Study the drawing (mm; zero at the part's minimum x, y, z) and answer. A direction names the side the tool comes from. Coordinates: 2 decimals unless noted, no trailing zeros. Loops run counter-clockwise (first coordinate to the right, second up) from the corner with the lowest first, then second, coordinate; pieces in that order, holes last. Notation, with made-up numbers: (70.5, 18) - (75.5, 18) arc R16 ccw to (75.5, 29) - close; hole circle Ø4 at (88, 33). An arc over 180 degrees is marked (long way). Use one line per item in the form item = value.
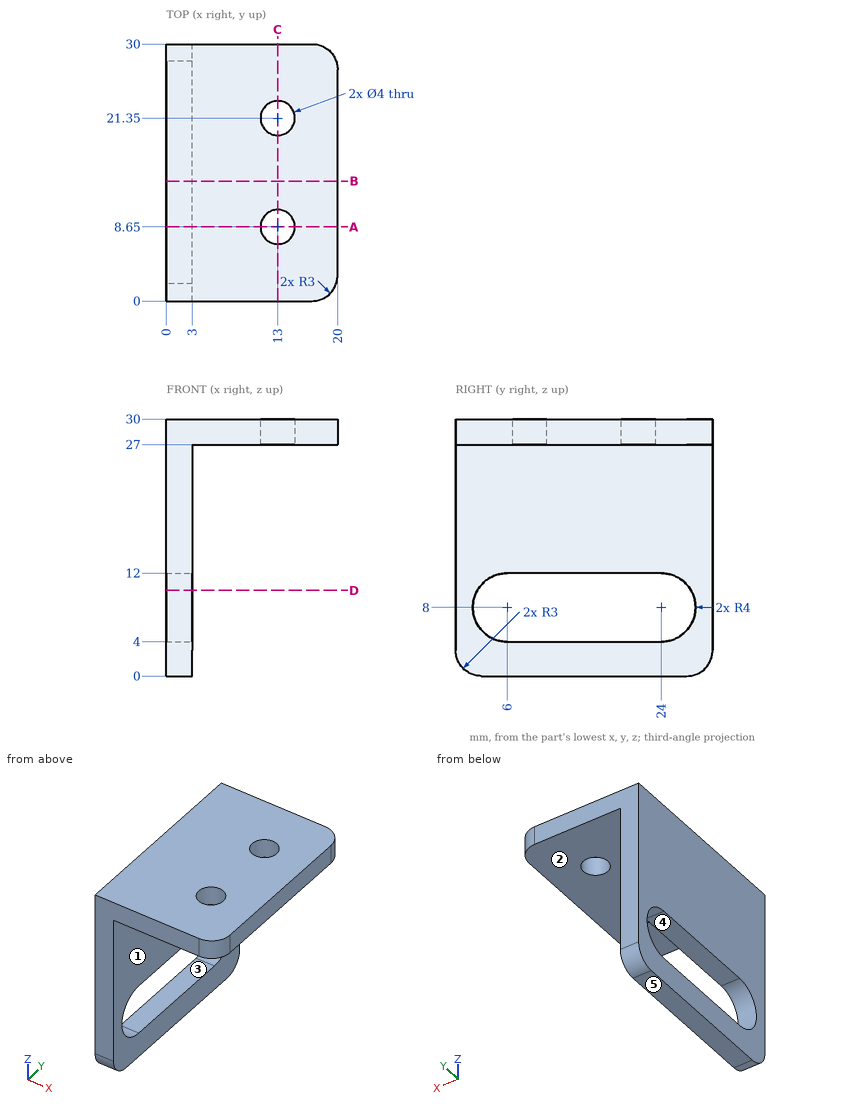
Item 1: The part is cut by section A-A on y = 8.65. Give the vertices of the cut face in (x, z), plus the area to 3 significant figures.
Results below:
outline = (0, 0) - (3, 0) - (3, 4) - (0, 4) - close; (0, 12) - (3, 12) - (3, 27) - (11, 27) - (11, 30) - (0, 30) - close; (15, 27) - (20, 27) - (20, 30) - (15, 30) - close
area = 105 mm²
Item 2: Which of the six approach directions +Z, -Z, +X, -X, +Y, -Y give full straight-line access (tool end or side, diameter ignored) to the marked faces 4 and 5?
Results below:
face_4 = +X, -X
face_5 = -Z, +X, -X, +Y, -Y
Item 3: The part is cut by section D-D on z = 10. Give the vertices of the cut face in (x, y), plus the area to 3 significant figures.
Results below:
outline = (0, 0) - (3, 0) - (3, 2.54) - (0, 2.54) - close; (0, 27.46) - (3, 27.46) - (3, 30) - (0, 30) - close
area = 15.2 mm²
Item 4: The part is cut by section B-B on y = 14. Give the vertices of the cut face in (x, z), plus the area to 3 significant figures.
Results below:
outline = (0, 0) - (3, 0) - (3, 4) - (0, 4) - close; (0, 12) - (3, 12) - (3, 27) - (20, 27) - (20, 30) - (0, 30) - close
area = 117 mm²
Item 5: The part is cut by section C-C on x = 13. Give the vertices of the cut face in (y, z), plus the area to 3 significant figures.
Results below:
outline = (0, 27) - (6.65, 27) - (6.65, 30) - (0, 30) - close; (10.65, 27) - (19.35, 27) - (19.35, 30) - (10.65, 30) - close; (23.35, 27) - (30, 27) - (30, 30) - (23.35, 30) - close
area = 66.0 mm²
Item 6: Find the intervals of material crossed by L1, parallel to Y at x = 13, z = 28.6; L2, parallel to X at y = 5, z = 20.75; L3, parallel to Z at x = 16.5, y = 25.25, in increasing order.
Results below:
L1 = 0 to 6.65, 10.65 to 19.35, 23.35 to 30
L2 = 0 to 3
L3 = 27 to 30
Item 7: For a pull along Z with two mould halves and no side action, classify the marked faces 1, 2 and 3 as +Z half, -Z half, draft (parallel to the pull), parting line (faces both ways), or undercut.
Results below:
face_1 = draft
face_2 = -Z half
face_3 = undercut
Item 8: Each of these flat-tipped pins is pushed along its axis until it touches: P1, Ø5, axis at y = 23.5, z = 13.5, coming from the +X side; P2, Ø1.5, axis at x = 15, y = 16.5, coming from the -Z side; P3, Ø12, axis at x = 8.5, y = 20, coming from the -Z side. Where does it stop, or does it pass through?
Results below:
P1 = 3
P2 = 27
P3 = 0
